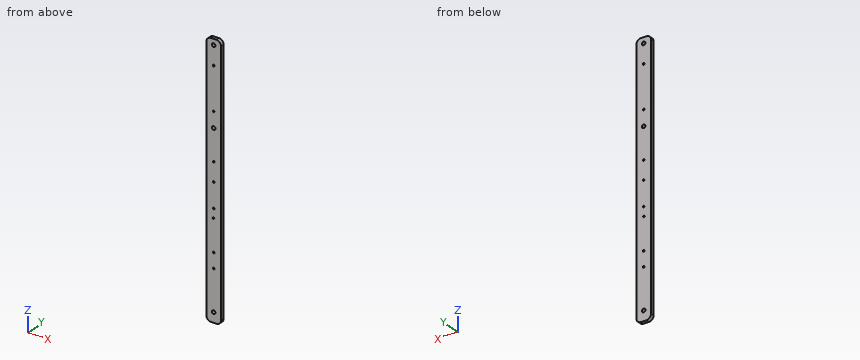
```python
from build123d import *

# Parameters (mm, degrees)
F0_R     = 3
F0_R_2   = 1.5
F1_DEPTH = 6.35


with BuildPart() as f1:
    # F0 (on Front) → F1 (new body)
    with BuildSketch(Plane.XZ):
        with BuildLine():
            ThreePointArc((-12.7, -188.950539), (-10.352556, -194.61777), (-4.685325, -196.965214))
            Line((-4.685325, -196.965214), (4.685325, -196.965214))
            ThreePointArc((4.685325, -196.965214), (10.352556, -194.61777), (12.7, -188.950539))
            Line((12.7, -188.950539), (12.7, 245.383261))
            ThreePointArc((12.7, 245.383261), (10.352556, 251.050492), (4.685325, 253.397937))
            Line((4.685325, 253.397937), (0, 253.397937))
            Line((0, 253.397937), (-4.685325, 253.397937))
            ThreePointArc((-4.685325, 253.397937), (-10.352556, 251.050492), (-12.7, 245.383261))
            Line((-12.7, 245.383261), (-12.7, -188.950539))
        make_face()
        with Locations((0, -180.083141)):
            Circle(F0_R, mode=Mode.SUBTRACT)
        with Locations((0, -110.852026)):
            Circle(F0_R_2, mode=Mode.SUBTRACT)
        with Locations((0, -85.452026)):
            Circle(F0_R_2, mode=Mode.SUBTRACT)
        with Locations((-0.438477, -31.045226)):
            Circle(F0_R_2, mode=Mode.SUBTRACT)
        with Locations((0, -15.452026)):
            Circle(F0_R_2, mode=Mode.SUBTRACT)
        with Locations((0, 26.554786)):
            Circle(F0_R_2, mode=Mode.SUBTRACT)
        with BuildLine():
            ThreePointArc((1.5, 58.558786), (-1.06066, 57.498125), (0, 60.058786))
            ThreePointArc((0, 60.058786), (1.06066, 59.619446), (1.5, 58.558786))
        make_face(mode=Mode.SUBTRACT)
        with BuildLine():
            ThreePointArc((0, 109.087622), (-3, 112.087622), (0, 115.087622))
            ThreePointArc((0, 115.087622), (2.12132, 114.208943), (3, 112.087622))
            ThreePointArc((3, 112.087622), (2.12132, 109.966302), (0, 109.087622))
        make_face(mode=Mode.SUBTRACT)
        with BuildLine():
            ThreePointArc((0, 137.061597), (-1.5, 138.561597), (0, 140.061597))
            ThreePointArc((0, 140.061597), (1.06066, 139.622258), (1.5, 138.561597))
            ThreePointArc((1.5, 138.561597), (1.06066, 137.500937), (0, 137.061597))
        make_face(mode=Mode.SUBTRACT)
        with BuildLine():
            ThreePointArc((0, 209.458786), (-1.5, 210.958786), (0, 212.458786))
            ThreePointArc((0, 212.458786), (1.06066, 212.019446), (1.5, 210.958786))
            ThreePointArc((1.5, 210.958786), (1.06066, 209.898125), (0, 209.458786))
        make_face(mode=Mode.SUBTRACT)
        with BuildLine():
            ThreePointArc((0, 240.519919), (-3, 243.519919), (0, 246.519919))
            ThreePointArc((0, 246.519919), (2.12132, 245.64124), (3, 243.519919))
            ThreePointArc((3, 243.519919), (2.12132, 241.398599), (0, 240.519919))
        make_face(mode=Mode.SUBTRACT)
    extrude(amount=F1_DEPTH)


solid = f1.part
```
Part model, mm, in its own coordinate system. Round coordinates to 2 decimals unless told otherwise and drop trailing zeros. Answer in a Markdown table with one row per item. Add a question column.
Q1. Pin check, flat tips, straight feed: pin 1 (2.5 mm diameter, centred on x = 0, z = -85.45, fed in from -Y); pin 2 (4 mm diameter, centred on x = 0, z = -110.85, fed in from -Y). Stop position of each tip, or through.
Q2. Wall check: L1, parallel to Z at x = 2, y = -4.25; L2, parallel to X at y = -2.5, z = 59; L3, parallel to Z at x = -5.75, y = -3. Give the ranges that are in metal, low to high. Write a range as from..to.
Q3. Cut at A-A on y = -2.25. Give the number of separate pieces and of enclosed holes in the cut face, and give its area (3 significant figures).
Established:
| question | item | result |
|---|---|---|
| 1 | pin 1 | passes through |
| 1 | pin 2 | stops at y = -6.35 |
| 2 | L1 | z = -196.97..-182.32, -177.85..109.85, 114.32..241.28, 245.76..253.4 |
| 2 | L2 | x = -12.7..-1.43, 1.43..12.7 |
| 2 | L3 | z = -196.89..253.33 |
| 3 | separate pieces | 1 |
| 3 | enclosed holes | 11 |
| 3 | area | 11,200 mm2 |
